Design review of the part built by this model. Coordinates are the model's own, in mm. A direction names the side the tool comes from. Give positions to 0.01 mm unless a question says otherwise; leave off trailing zeros. Loops run counter-clockwise (first coordinate to the right, second up) from the corner with the lowest first, then second, coordinate; pieces in that order, holes last. Notation, with made-up numbers: (64, 83.25) - (105, 83.25) arc R7 ccw to (105, 90.25) - close; hole circle Ø6 at (16, -22). An arc over 180 degrees is marked (long way). Write each question's results on one line, items separated by ' | '.
```python
from build123d import *

# Parameters (mm, degrees)
F0_W     = 100
F0_H     = 70
F0_R     = 6
F1_DEPTH = 20
F2_R     = 40
F3_R     = 1.5
F4_DEPTH = 25


with BuildPart() as f1:
    # F0 (on Top) → F1 (new body, symmetric)
    with BuildSketch(Plane.XY):
        with Locations((0, 35)):
            Rectangle(F0_W, F0_H)
        with Locations((0, 50)):
            Circle(F0_R, mode=Mode.SUBTRACT)
    extrude(amount=F1_DEPTH, both=True)

    # F2
    f2_edges = [f1.edges().sort_by_distance(p)[0] for p in [
        (-50, 70, 0),
        (50, 70, 0),
    ]]
    fillet(f2_edges, radius=F2_R)

    # F3 (on face) → F4 (cut)
    with BuildSketch(Plane.XZ):
        with Locations((-30, 10)):
            Circle(F3_R)
        with Locations((-30, -10)):
            Circle(F3_R)
        with Locations((30, -10)):
            Circle(F3_R)
        with Locations((30, 10)):
            Circle(F3_R)
    extrude(amount=-F4_DEPTH, mode=Mode.SUBTRACT)


solid = f1.part
```
Item 1: We need section B-B on x = 0. Give the boundary of the cut face in (y, z).
Output values:
outline: (0, -20) - (44, -20) - (44, 20) - (0, 20) - close; (56, -20) - (70, -20) - (70, 20) - (56, 20) - close
Item 2: We need section D-D on z = -15. Give the boundary of the cut face in (x, y).
Output values:
outline: (-50, 0) - (50, 0) - (50, 30) arc R40 ccw to (10, 70) - (-10, 70) arc R40 ccw to (-50, 30) - close; hole circle Ø12 at (0, 50)
Item 3: Draft analysis for pull direction Z (two halves, no side actions). For faces 1 (the face through (-1, 35, -20)), 2 (the face through (-1, 35, 20)), 3 (the face through (50, 15, 0)), 4 (the face through (-30, 25, 10)), state which applies: +Z half, -Z half, draft (parallel to the pull), parting line (faces both ways), or undercut.
Output values:
face 1: -Z half | face 2: +Z half | face 3: draft | face 4: undercut
Item 4: We need section A-A on z = 10. Give the boundary of the cut face in (x, y).
Output values:
outline: (-50, 0) - (-31.5, 0) - (-31.5, 25) - (-28.5, 25) - (-28.5, 0) - (28.5, 0) - (28.5, 25) - (31.5, 25) - (31.5, 0) - (50, 0) - (50, 30) arc R40 ccw to (10, 70) - (-10, 70) arc R40 ccw to (-50, 30) - close; hole circle Ø12 at (0, 50)
Item 5: We need section C-C on y = 45.5. Give the boundary of the cut face in (x, z), then the cut area to 3 significant figures.
Output values:
outline: (-46.87, -20) - (-3.97, -20) - (-3.97, 20) - (-46.87, 20) - close; (3.97, -20) - (46.87, -20) - (46.87, 20) - (3.97, 20) - close | area: 3,430 mm²
Item 6: Wall thickness on probe 1 along Z at (x, y) = (30, 10.75); probe 2 along Y at (x, z) = (0, -1); probe 3 along X at (y, z) = (31, 17.5): over which ranges is each line inside the solid? List them lowest first.
Output values:
probe 1: z = -20 to -11.5, -8.5 to 8.5, 11.5 to 20 | probe 2: y = 0 to 44, 56 to 70 | probe 3: x = -49.99 to 49.99
Item 7: Clearance check with flat-ended pins moving along their axes: P1, Ø5, axis at x = -30, z = 10, coming from the +Y side; P2, Ø2.5, axis at x = 30, z = -10.5, coming from the -Y side; P3, Ø4, axis at y = 42.5, z = 5, coming from the +X side; P4, Ø1, axis at x = -20, z = 1.5, coming from the +Y side. State where each tip first meets the part, or that it passes through.
Output values:
P1: stops at y = 65.97 | P2: stops at y = 0 | P3: stops at x = 48.6 | P4: stops at y = 68.86
Item 8: Tool access review of faces 5 (the face through (-31.5, 12.32, -9.93)), 6 (the face through (38.594, 57.972, -0.28)): name each direction out of +Z, -Z, +X, -X, +Y, -Y from which nothing blocks a thin tool from reaching the whole face with its end or side.
Output values:
face 5: -Y | face 6: +Z, -Z, +X, +Y
